For this review, take the finished solid that the model builds, in its own axes (mm). A direction names the side the tool comes from. Coordinates: 2 decimals unless noted, no trailing zeros. Order: outer loops, then holes, each group sorted by start corner. A loop starts at its lowest first (then second) coordinate and runs counter-clockwise, first axis right, second up. Notation, with made-up numbers: M 64,80 L 82,80 A5 ccw 82,87 Z; hole C -14.75,30.5 d5. An arc over 180 degrees is marked long. Use one line per item in the form item = value. Start each with the question number.
Autodesk Inventor part; units mm, degrees
ref_plane "YZ Plane" through (0, 0, 0) normal (1, 0, 0) x (0, 1, 0)
ref_plane "XZ Plane" through (0, 0, 0) normal (0, 1, 0) x (-1, 0, 0)
ref_plane "XY Plane" through (0, 0, 0) normal (0, 0, 1) x (1, 0, 0)
sketch "Эскиз2" plane through (0, 0, 0) normal (1, 0, 0) x (0, 1, 0)
  line L0 (0, 0) -> (-3, 0)
  line L1 (-3, 0) -> (-3, 36)
  line L2 (-3, 36) -> (0, 36)
  line L3 (0, 36) -> (0, 0)
  line L4 (-3, 0) -> (0, 0)
  line L5 (0, 0) -> (0, -5)
  line L6 (0, -5) -> (-3, -5)
  line L7 (-3, -5) -> (-3, 0)
  line L8 (-3, 36) -> (0, 36)
  line L9 (0, 36) -> (0, 41)
  line L10 (0, 41) -> (-3, 41)
  line L11 (-3, 41) -> (-3, 36)
  line L12 (0, 0) -> (0, 36)
  line L13 (0, 36) -> (0, 34)
  line L14 (0, 0) -> (0, 2)
  line L15 (29.146, 18) -> (29.146, 26)
  line L16 (29.146, 26) -> (29.146, 10)
  line L17 (29.146, 10) -> (0, 2)
  line L18 (29.146, 26) -> (0, 34)
  point P0 (19.146, 0)
  dimension "d4" = 3
  dimension "d5" = 36
  dimension "d6" = 5
  dimension "d7" = 5
  dimension "d8" = 19.146
  dimension "d13" = 2
  dimension "d14" = 2
extrude "Выдавливание2" add sketch "Эскиз2" along normal blind 3
sketch "Эскиз3" plane through (3, 0, 0) normal (1, 0, 0) x (0, 0, -1)
  line L0 (5, -3) -> (5, 0)
  line L1 (5, 0) -> (-41, 0)
  line L2 (5, -3) -> (-41, -3)
  line L3 (-41, -3) -> (-41, 0)
  line L4 (-41, 0) -> (5, 0)
  line L5 (5, 0) -> (5, -3)
  point P0 (0, 0)
  point P1 (-34, 0)
extrude "Выдавливание3" add sketch "Эскиз3" along normal blind 25
sketch "Эскиз5" plane through (0, 0, 2) normal (0, 1, 0) x (1, 0, 0)
  line L0 (0, 7) -> (28, 7)
  line L1 (0, 7) -> (0, 2)
  line L2 (0, 7) -> (0, 0)
  line L3 (0, 2) -> (28, 2)
  line L4 (28, -39) -> (28, 7)
  line L5 (0, 7) -> (0, -39)
  line L6 (0, -39) -> (0, -34)
  line L7 (0, -34) -> (28, -34)
  line L8 (28, -34) -> (21, -34)
  line L9 (21, -34) -> (7, -34)
  line L10 (7, -34) -> (7, 2)
  circle A0 centre (7, -34) radius 1.6
  circle A1 centre (21, -34) radius 1.6
  circle A2 centre (7, 2) radius 1.6
  circle A3 centre (21, 2) radius 1.6
  point P0 (0, -32)
  dimension "d17" = 5
  dimension "d18" = 7
  dimension "d19" = 14
  dimension "d20" = 3.2
  dimension "d21" = 3.2
  dimension "d22" = 3.2
  dimension "d23" = 3.2
extrude "Выдавливание4" cut sketch "Эскиз5" against normal blind 25 contours A2 L3 | L3 L10 A2 | A3 L3 | L3 A3 | L3 A2 L10 | A1 L7 | L7 A1 | A0 L10 L7 | L7 A0 | A0 L7 L10
sketch "Эскиз7" plane through (3, 0, 0) normal (1, 0, 0) x (0, 0, -1)
  line L0 (-10, 29.146) -> (-26, 29.146)
  line L1 (-26, 29.146) -> (-10, 29.146)
  line L2 (-10, 29.146) -> (-10, 26.146)
  line L3 (-10, 26.146) -> (-26, 26.146)
  line L4 (-26, 26.146) -> (-26, 29.146)
  point P0 (0, 0)
  dimension "d37" = 3
extrude "Выдавливание6" add sketch "Эскиз7" along normal blind 155 and the other way blind 3
sketch "Эскиз8" plane through (0, 29.146, 26) normal (0, 1, 0) x (1, 0, 0)
  line L0 (158, 16) -> (158, 0)
  line L1 (0, -15) -> (0, 31)
  line L2 (158, 16) -> (0, 16)
  line L3 (0, 16) -> (0, 13)
  line L4 (0, 13) -> (158, 13)
  line L5 (158, 13) -> (158, 16)
  line L6 (0, 0) -> (3, 0)
  line L7 (0, 0) -> (158, 0)
  line L8 (158, 0) -> (158, 3)
  line L9 (158, 3) -> (0, 3)
  line L10 (0, 3) -> (0, 0)
  point P0 (0, 26)
  point P1 (158, 3)
  point P2 (0, 3)
  dimension "d38" = 3
  dimension "d39" = 3
extrude "Выдавливание7" add sketch "Эскиз8" along normal blind 11 contours L0 L4 L1 L2 | L0 L7 L6 L1 L9
sketch "Эскиз9" plane through (3, 0, 0) normal (1, 0, 0) x (0, 0, -1)
  line L0 (-26, 29.146) -> (-34, 0)
  line L1 (-34, 0) -> (-26, 29.146)
  line L2 (-26, 29.146) -> (-10, 29.146)
  line L3 (-10, 29.146) -> (-2.177, 0)
  line L4 (-2.177, 0) -> (-34, 0)
  line L5 (-1.6, 0) -> (1.6, 0)
  line L6 (-26, 29.146) -> (-23.107, 28.3519)
  line L7 (-23.107, 28.3519) -> (-30.889, 0)
  line L8 (-2, 0) -> (-10, 29.146)
  line L9 (-2, 0) -> (-5.111, 0)
  line L10 (-34, 0) -> (-2, 0)
  line L11 (-10, 29.146) -> (-12.8975, 28.3685)
  line L12 (-10, 29.146) -> (-7, 29.146) construction
  line L13 (-12.8975, 28.3685) -> (-5.111, 0)
  point P0 (0, 0)
  dimension "d42" = 3
  dimension "d43" = 3.111
  dimension "d44" = 3
  dimension "d45" = 164.98
extrude "Выдавливание8" add sketch "Эскиз9" along normal blind 25 contours L6 L7 L4 L0 | L3 L4 L13 L11
sketch "Эскиз10" plane through (0, 40.146, 26) normal (0, 1, 0) x (1, 0, 0)
  line L0 (0, 0) -> (0, -8)
  line L1 (158, 16) -> (28, 16)
  line L2 (0, 0) -> (158, 0)
  line L3 (158, 0) -> (158, 16)
  line L4 (158, 16) -> (0, 16)
  line L5 (0, 16) -> (0, 0)
  line L6 (0, -15) -> (0, 31)
  line L7 (0, 8) -> (0, 10.5)
  line L8 (0, 10.5) -> (0, 5.5)
  line L9 (0, 5.5) -> (158, 5.5)
  line L10 (158, 13) -> (158, 3)
  line L11 (158, 5.5) -> (158, 10.5)
  line L12 (158, 10.5) -> (0, 10.5)
  line L13 (0, 13) -> (158, 13)
  point P0 (0, 26)
  point P1 (28, 16)
  dimension "d48" = 2.5
  dimension "d49" = 5
extrude "Выдавливание9" add sketch "Эскиз10" along normal blind 2 contours L3 L13 L5 L4 L1 | L3 L12 L5 L13 | L3 L2 L5 L9
sketch "Эскиз11" plane through (28, 26.146, 10) normal (0, -1, 0) x (1, 0, 0)
  line L0 (130, 0) -> (-28, 0)
  line L1 (130, 0) -> (130, -10)
  line L2 (125, -5) -> (125, 21)
  line L3 (130, 16) -> (130, 10.5)
  line L4 (130, 21) -> (130, 16)
  line L5 (130, 16) -> (130, 21)
  line L6 (130, 21) -> (130, 26)
  line L7 (130, 26) -> (120, 26)
  line L8 (120, 26) -> (120, -10)
  line L9 (120, -10) -> (130, -10)
  line L10 (-28, 16) -> (130, 16)
  line L11 (51, 16) -> (120, 26)
  line L12 (120, -10) -> (51, 0)
  circle A0 centre (125, 21) radius 1.6
  circle A1 centre (125, -5) radius 1.6
  point P0 (-28, -10)
  dimension "d52" = 10
  dimension "d54" = 26
  dimension "d56" = 10
  dimension "d57" = 3.2
  dimension "d58" = 3.2
extrude "Выдавливание10" add sketch "Эскиз11" against normal blind 3 contours L1 L9 L8 L0 | L8 L12 L0 | L10 L8 L7 L6 L4 | L10 L11 L8
fillet "Сопряжение1" radius 4 4 edges at (158, 27.646, 36) (158, 27.646, 0) (148, 27.646, 0) (148, 27.646, 36)
fillet "Сопряжение2" radius 100 2 edges at (79, 27.646, 10) (79, 27.646, 26)
properties part number "reyka"
1. For pin 1 Ø10 at (y, z) = (8.5, 15.5) entering from +X; pin 2 Ø4 at (x, z) = (153, 5) entering from -Y; pin 3 Ø4 at (x, y) = (69.5, 37.5) entering from +Z; pin 4 Ø6 at (x, y) = (77.5, 20.5) entering from -Z, all flat-tipped, find the tip position at first contact; note any pin that passes through.
2. Consider section C-C, the plane x = 41. Write out the cut boundary in (y, z).
3. Consider section B-B, the plane y = 34. Write out the cut boundary in (x, z), plus the area to 3 significant figures.
4. The part is to be moulded in two halves that separate along Z. For faces 1 (the flat face through (3, 10, 18)), 2 (the flat face through (14, -3, 18)), 3 (the flat face through (116.493, 27.625, 31.434)), say which applies: pulls with the +Z half, pulls with the -Z half, needs draft (parallel to the pull), parting line crosses it, or undercut.
5. Tool access review of faces 4 (the flat face through (15, 0, 18)), 5 (the cylindrical face through (78.88, 27.67, 9.75)), 6 (the flat face through (80, 35, 23)), 7 (the flat face through (133, 29.146, 6)): name each direction out of +Z, -Z, +X, -X, +Y, -Y from which nothing blocks a thin tool from reaching the whole face with its end or side.
6. To check wall thickness, follow line 1 (Z direction, x = 7, y = -0.7); line 2 (Z direction, x = 153, y = 27.9); line 3 (X direction, y = -0.6, z = 36). State the ranges of each line that lie inside material, in increasing order.
7. Consider section A-A, the plane x = 7. Give the number of separate pieces and of enclosed holes in the cut face, plus the area to 3 significant figures.
8. Consider section D-D, the plane y = 14. Write out the cut boundary in (x, z).
Answers follow:
q1.pin_1 = 3
q1.pin_2 = 26.15
q1.pin_3 = 26
q1.pin_4 = through
q2.outline = M 26.15,10 L 42.15,10 L 42.15,15.5 L 40.15,15.5 L 40.15,13 L 29.15,13 L 29.15,23 L 40.15,23 L 40.15,20.5 L 42.15,20.5 L 42.15,26 L 26.15,26 Z
q3.outline = M 0,10 L 158,10 L 158,13 L 0,13 Z; M 0,23 L 158,23 L 158,26 L 0,26 Z
q3.area = 948 mm²
q4.face_1 = undercut
q4.face_2 = needs draft
q4.face_3 = pulls with the +Z half
q5.face_4 = +X
q5.face_5 = -Z, +Y, -Y
q5.face_6 = +X, -X
q5.face_7 = -Z, +X, -X, +Y
q6.line_1 = -5 to -1.6, 1.6 to 34.4, 37.6 to 41
q6.line_2 = 0 to 3.4, 6.6 to 29.4, 32.6 to 36
q6.line_3 = 0 to 5.4, 8.6 to 19.4, 22.6 to 28
q7.separate_pieces = 3
q7.enclosed_holes = 1
q7.area = 417 mm²
q8.outline = M 0,5.84 L 3,5.84 L 3,5.93 L 28,5.93 L 28,8.95 L 3,8.95 L 3,27.05 L 28,27.05 L 28,30.16 L 0,30.16 Z
